Verification items for the finished model (mm, model axes). A direction names the side the tool comes from. Round coordinates to 2 decimals unless told otherwise and drop trailing zeros. Order: outer loops, then holes, each group sorted by start corner. A loop starts at its lowest first (then second) coordinate and runs counter-clockwise, first axis right, second up. Notation, with made-up numbers: (32.5, -22.75) -> (77.5, -22.75) arc R22 cw to (77.5, -6.75) -> close; hole circle Ø5 at (-1.5, -32). An arc over 180 degrees is marked (long way). Return JSON: item names as keys, results as strings. Group by question number.
1) Tool access check on faces 1 (the flat face through (-10, 0, -9)), 2 (the flat face through (-7, 0.7, -11.5)). Record the directions out of +Z, -Z, +X, -X, +Y, -Y that give a thin tool (end or side, any length) a straight path to the whole face; none if there is none.
2) Section check A-A on x = -9. Enter the section's corners in (y, z).
3) Scan line: L1, parallel to Z at x = -8.5, y = 0.45. Record every from-to range of solid material in increasing order.
4) Draft check along Z on faces 3 (the flat face through (-10, 1, 0)), 4 (the flat face through (-10, 1.5, -9)), 5 (the flat face through (-10, 1, -11)). Enter one of: pulls with the +Z half, pulls with the -Z half, needs draft (parallel to the pull), parting line crosses it, or undercut.
Autodesk Inventor part; units mm, degrees
ref_plane "YZ Plane" through (0, 0, 0) normal (1, 0, 0) x (0, 1, 0)
ref_plane "XZ Plane" through (0, 0, 0) normal (0, 1, 0) x (-1, 0, 0)
ref_plane "XY Plane" through (0, 0, 0) normal (0, 0, 1) x (1, 0, 0)
sketch "Sketch1" plane through (0, 0, 0) normal (0, 1, 0) x (-1, 0, 0)
  line L0 (0, 0) -> (0, -23)
  line L1 (0, -23) -> (20, -23)
  line L2 (20, -23) -> (20, 0)
  line L3 (16.0214, -11.5) -> (3.8301, -11.5) construction
  line L4 (20, 0) -> (0, 0)
  line L5 (13, -11) -> (7, -11)
  line L6 (7, -11) -> (7, -12)
  line L7 (7, -12) -> (13, -12)
  line L8 (13, -12) -> (13, -11)
  line L9 (10, -8) -> (10, -15) construction
  dimension "d0" = 23
  dimension "d10" = 20
  dimension "d13" = 10
  dimension "d14" = 1
  dimension "d15" = 6
extrude "Extrusion4" add sketch "Sketch1" along normal blind 1.5
properties part number "Distance_test_adaptor_slit_1mm"
Check result:
{
 "1": {"face 1": "+Z, -Z, +X, -X, -Y", "face 2": "+Y, -Y"},
 "2": {"outline": "(0, -23) -> (1.5, -23) -> (1.5, -12) -> (0, -12) -> close; (0, -11) -> (1.5, -11) -> (1.5, 0) -> (0, 0) -> close"},
 "3": {"L1": "-23 to -12, -11 to 0"},
 "4": {"face 3": "pulls with the +Z half", "face 4": "needs draft", "face 5": "undercut"}
}
